Can you work these out from the model? Positions are in its coordinate system, mm. Face numbers are marked on the shaded views. A direction names the side the tool comes from. Give positions to 0.01 mm unless a question says otherwise; leave off trailing zeros. Loops run counter-clockwise (first coordinate to the right, second up) from the corner with the lowest first, then second, coordinate; pieces in that order, holes last. Notation, with made-up numbers: (57.5, 54.5) -> (67.5, 54.5) arc R17 ccw to (67.5, 84.5) -> close; hole circle Ø1 at (69, 50.25). An arc over 180 degrees is marked (long way). One line per question, with ' | ' between items.
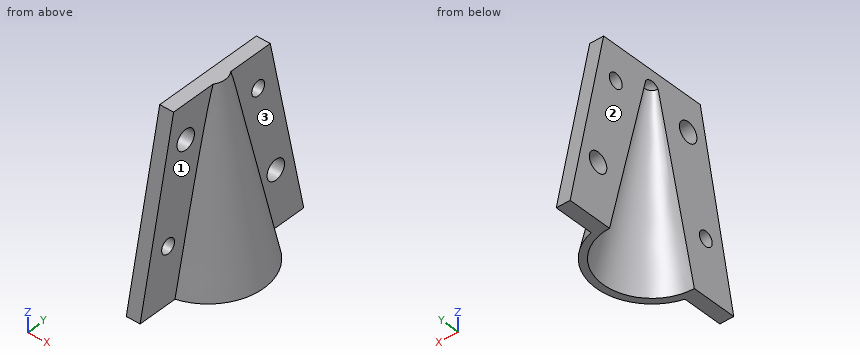
from build123d import *

# Parameters (mm, degrees)
SKETCH1_R                   = 8.89
BOSS_EXTRUDE1_DEPTH         = 30.48
BOSS_EXTRUDE1_TAPER         = 14
DOME1_FACE_RADIUS           = 1.290482473
DOME1_HEIGHT                = 0.635
BOSS_EXTRUDE2_DEPTH         = 33.02
DRAFT1_ANGLE                = -12
F_27_0_144_DIAMETER_HOLE1_D = 3.6576
F_6_32_TAPPED_HOLE1_D       = 2.7051
F_6_32_TAPPED_HOLE1_DEPTH   = 11.176
F_6_32_TAPPED_HOLE1_TIP     = 0.81269403
SKETCH12_W                  = 10.592126778
SKETCH12_H                  = 34.29
CUT_EXTRUDE1_DEPTH          = 39.568082983


with BuildPart() as part:
    # Sketch1 → Boss-Extrude1 (new body)
    with BuildSketch(Plane.XY):
        Circle(SKETCH1_R)
    extrude(amount=BOSS_EXTRUDE1_DEPTH, taper=BOSS_EXTRUDE1_TAPER)

    # Dome1: a dome of height H over a round flat face of radius A is a cap of a sphere of radius (A * A + H * H) / (2 * H)
    dome1_r = (DOME1_FACE_RADIUS * DOME1_FACE_RADIUS + DOME1_HEIGHT * DOME1_HEIGHT) / (2 * DOME1_HEIGHT)
    dome1_base = Plane((0, 0, 30.48), z_dir=(0, 0, 1))
    with Locations(dome1_base.offset(DOME1_HEIGHT - dome1_r)):
        dome1_ball = Sphere(dome1_r, mode=Mode.PRIVATE)
    add(split(dome1_ball, bisect_by=dome1_base, keep=Keep.TOP, mode=Mode.PRIVATE))


with BuildPart() as body_2:
    # Sketch2 → Boss-Extrude2 (new body)
    with BuildSketch(Plane.XY):
        with BuildLine():
            Line((-2.54, 17.145), (-2.54, 9.837377699))
            ThreePointArc((-2.54, 9.837377699), (-10.16, 0), (-2.54, -9.837377699))
            Line((-2.54, -9.837377699), (-2.54, -17.145))
            Line((-2.54, -17.145), (2.54, -17.145))
            Line((2.54, -17.145), (2.54, -9.837377699))
            ThreePointArc((2.54, -9.837377699), (10.16, 0), (2.54, 9.837377699))
            Line((2.54, 9.837377699), (2.54, 17.145))
            Line((2.54, 17.145), (-2.54, 17.145))
        make_face()
    extrude(amount=BOSS_EXTRUDE2_DEPTH)

    # Combine1: read off the stored shape, not the designer's step
    # Combine1: cut part
    add(part.part, mode=Mode.SUBTRACT)

    # Draft1
    draft1_faces = [body_2.faces().sort_by_distance(p)[0] for p in [
        (0, -17.145, 16.51),
        (0, 17.145, 16.51),
        (10.16, 0, 16.51),
        (-10.16, 0, 16.51),
    ]]
    draft(draft1_faces, Plane(origin=(0, 0, 0), x_dir=(-1, 0, 0), z_dir=(0, 0, -1)), DRAFT1_ANGLE)

    # #27 (0.144) Diameter Hole1 (through all)
    with Locations(Plane.ZY.offset(2.54)):
        with Locations((10.16, 11.285999498), (26.67, -7.590126179)):
            Hole(F_27_0_144_DIAMETER_HOLE1_D / 2)

    # #6-32 Tapped Hole1
    with Locations(Plane.ZY.offset(2.54)):
        with Locations((26.67, 7.590126179), (10.16, -11.285999498)):
            Hole(F_6_32_TAPPED_HOLE1_D / 2, depth=F_6_32_TAPPED_HOLE1_DEPTH)
            with Locations((0, 0, -(F_6_32_TAPPED_HOLE1_DEPTH + F_6_32_TAPPED_HOLE1_TIP / 2))):  # 118° drill point
                Cone(0, F_6_32_TAPPED_HOLE1_D / 2, F_6_32_TAPPED_HOLE1_TIP, mode=Mode.SUBTRACT)

    # Sketch12 → Cut-Extrude1 (cut, through all)
    with BuildSketch(Plane(origin=(0, 0, 0), x_dir=(-1, 0, 0), z_dir=(0, 0, -1))):
        with Locations((5.296063389, 0)):
            Rectangle(SKETCH12_W, SKETCH12_H)
    extrude(amount=-CUT_EXTRUDE1_DEPTH, mode=Mode.SUBTRACT)


solid = body_2.part
Q1. If we section it at C-C (z = 5.5): Write out the boundary of the cut face in (x, y).
Entries:
outline: (0, -15.98) -> (2.54, -15.98) -> (2.54, -8.62) arc R8.99 ccw to (2.54, 8.62) -> (2.54, 15.98) -> (0, 15.98) -> (0, 7.52) arc R7.52 cw to (0, -7.52) -> close
Q2. On a 3-axis mill with a long thin cutter (end or side, diameter ignored), from which of +Z, -Z, +X, -X, +Y, -Y can I reach the whole of each face in a straight line? I mean the marked faces 1, 2 and 3. Say none if no direction works.
Entries:
face 1: +Z, +X, -Y | face 2: +Z, -Z, -X, +Y, -Y | face 3: +Z, +X, +Y
Q3. If we section it at D-D (z = 10.16): Write out the boundary of the cut face in (x, y).
Entries:
outline: (0, -14.99) -> (2.54, -14.99) -> (2.54, -12.64) -> (0, -12.64) -> close; (0, -9.93) -> (2.54, -9.93) -> (2.54, -7.59) arc R8 ccw to (2.54, 7.59) -> (2.54, 9.46) -> (0, 9.46) -> (0, 6.36) arc R6.36 cw to (0, -6.36) -> close; (0, 13.11) -> (2.54, 13.11) -> (2.54, 14.99) -> (0, 14.99) -> close
Q4. If we section it at A-A (z = 26.67): Write out the boundary of the cut face in (x, y), plus the area to 3 significant figures.
Entries:
outline: (0, -11.48) -> (2.54, -11.48) -> (2.54, -9.42) -> (0, -9.42) -> close; (0, -5.76) -> (2.54, -5.76) -> (2.54, -3.7) arc R4.49 ccw to (2.54, 3.7) -> (2.54, 6.24) -> (0, 6.24) -> (0, 2.24) arc R2.24 cw to (0, -2.24) -> close; (0, 8.94) -> (2.54, 8.94) -> (2.54, 11.48) -> (0, 11.48) -> close | area: 44.4 mm²
Q5. If we section it at B-B (y = 0): Write out the boundary of the cut face in (x, z) (3 decimals), plus the area to 3 significant figures.
Entries:
outline: (0, 31.115) arc R1.629 cw to (1.29, 30.48) -> (8.89, 0) -> (10.16, 0) -> (3.141, 33.02) -> (0, 33.02) -> close | area: 63.9 mm²
Q6. For pin 1 Ø8 at (y, z) = (-10, 5.5) entering from +X; pin 2 Ø6 at (y, z) = (-1, 6) entering from +X; pin 3 Ø1.5 at (y, z) = (-1.5, 21.5) entering from +X, each with a flat end and sliding along its axis, tell me the tip position at first contact or that it passes through.
Entries:
pin 1: x = 6.87 | pin 2: x = 9.5 | pin 3: x = 5.62
Q7. If I drill on probe 1 along Y at (x, z) = (0.9, 26.67); probe 2 along X at (y, z) = (7, 28); probe 3 along Y at (x, z) = (1.15, 26.67), over which ranges is the centre line in solid material (lowest first)? Write a range as from..to.
Entries:
probe 1: -11.48..-9.42, -5.76..-2.05, 2.05..6.24, 8.94..11.48 | probe 2: 0..2.54 | probe 3: -11.48..-9.42, -5.76..-1.92, 1.92..6.24, 8.94..11.48
